Part model, mm, in its own coordinate system. A direction names the side the tool comes from. Coordinates: 2 decimals unless noted, no trailing zeros. Order: outer loops, then holes, each group sorted by start corner. A loop starts at its lowest first (then second) coordinate and runs counter-clockwise, first axis right, second up.
```python
from build123d import *

# Parameters (mm, degrees)
SKETCH1_W                 = 120
SKETCH1_H                 = 70
BOSS_EXTRUDE1_DEPTH       = 3
SKETCH6_W                 = 15
SKETCH6_H                 = 20
BOSS_EXTRUDE3_DEPTH       = 13
SKETCH7_W                 = 12.1
SKETCH7_H                 = 10.1
CUT_EXTRUDE3_DEPTH        = 71
SKETCH8_W                 = 15
SKETCH8_H                 = 4.3
BOSS_EXTRUDE4_DEPTH       = 2
SKETCH9_W                 = 1
SKETCH9_H                 = 6
CUT_EXTRUDE4_DEPTH        = 2
SKETCH10_W                = 3.5
SKETCH10_H                = 3
BOSS_EXTRUDE5_DEPTH       = 1.2
CHAMFER1_SIZE             = 1
CHAMFER1_OF_MIRROR3_SIZE  = 1
CUT_EXTRUDE5_REACH        = 18
SKETCH3_R                 = 1.625
SKETCH12_R                = 3
SKETCH12_R_2              = 1.625
BOSS_EXTRUDE7_DEPTH       = 4
CUT_EXTRUDE6_REACH        = 18
SKETCH11_R                = 1.625
SKETCH13_R                = 3
SKETCH13_R_2              = 1.625
BOSS_EXTRUDE8_DEPTH       = 4
SKETCH14_R                = 1.625
CUT_EXTRUDE7_DEPTH        = 4
SKETCH15_R                = 3.25
SKETCH15_R_2              = 1.625
SKETCH15_R_3              = 3
BOSS_EXTRUDE13_DEPTH      = 4
SKETCH17_W                = 5
SKETCH17_H                = 25
CUT_EXTRUDE8_DEPTH        = 4
SKETCH18_R                = 3
SKETCH18_R_2              = 1.625
BOSS_EXTRUDE14_DEPTH      = 4
FILLET2_R                 = 2
SKETCH19_R                = 1.625
CUT_EXTRUDE9_DEPTH        = 4
LPATTERN1_COUNT           = 2
LPATTERN1_PITCH           = 30
LPATTERN1_COL_COUNT       = 2
LPATTERN1_COL_PITCH       = 30
LPATTERN2_COUNT           = 4
LPATTERN2_PITCH           = 30
LPATTERN2_COPY_1_SKETCH_R = 1.625
LPATTERN2_COPY_1_DEPTH    = 4
LPATTERN2_COPY_2_SKETCH_R = 1.625
LPATTERN2_COPY_2_DEPTH    = 4
LPATTERN2_COPY_3_SKETCH_R = 1.625
LPATTERN2_COPY_3_DEPTH    = 4
LPATTERN2_COPY_4_SKETCH_R = 1.625
LPATTERN2_COPY_4_DEPTH    = 4
LPATTERN2_COPY_5_SKETCH_R = 1.625
LPATTERN2_COPY_5_DEPTH    = 4
LPATTERN2_COPY_6_SKETCH_R = 1.625
LPATTERN2_COPY_6_DEPTH    = 4


with BuildPart() as part:
    # Sketch1 → Boss-Extrude1 (new body)
    with BuildSketch(Plane(origin=(0, 0, 0), x_dir=(1, 0, 0), z_dir=(0, 1, 0))):
        Rectangle(SKETCH1_W, SKETCH1_H)
    extrude(amount=BOSS_EXTRUDE1_DEPTH)

    # Sketch6 → Boss-Extrude3 (add)
    with BuildSketch(Plane(origin=(0, 3, 0), x_dir=(1, 0, 0), z_dir=(0, 1, 0))):
        with Locations((-52.5, 25)):
            Rectangle(SKETCH6_W, SKETCH6_H)
        with Locations((-52.5, -25)):
            Rectangle(SKETCH6_W, SKETCH6_H)
    extrude(amount=BOSS_EXTRUDE3_DEPTH)

    # Sketch7 → Cut-Extrude3 (cut, through all)
    with BuildSketch(Plane(origin=(0, 0, -35), x_dir=(-1, 0, 0), z_dir=(0, 0, -1))):
        with Locations((52.55, 8.95)):
            Rectangle(SKETCH7_W, SKETCH7_H)
    extrude(amount=-CUT_EXTRUDE3_DEPTH, mode=Mode.SUBTRACT)

    # Sketch8 → Boss-Extrude4 (add)
    with BuildSketch(Plane(origin=(0, 3.9, 0), x_dir=(1, 0, 0), z_dir=(0, 1, 0))):
        with Locations((-52.5, -17.15)):
            Rectangle(SKETCH8_W, SKETCH8_H)
    boss_extrude4 = extrude(amount=BOSS_EXTRUDE4_DEPTH)

    # Mirror1: Boss-Extrude4 across plane
    add(boss_extrude4.mirror(Plane.XY))

    # Sketch9 → Cut-Extrude4 (cut)
    with BuildSketch(Plane(origin=(0, 16, 0), x_dir=(1, 0, 0), z_dir=(0, 1, 0))):
        with Locations((-54.75, 32)):
            Rectangle(SKETCH9_W, SKETCH9_H)
        with Locations((-50.25, 32)):
            Rectangle(SKETCH9_W, SKETCH9_H)
    cut_extrude4 = extrude(amount=-CUT_EXTRUDE4_DEPTH, mode=Mode.SUBTRACT)

    # Mirror2: Cut-Extrude4 across plane
    add(cut_extrude4.mirror(Plane.XY), mode=Mode.SUBTRACT)

    # Sketch10 → Boss-Extrude5 (add)
    with BuildSketch(Plane(origin=(0, 0, -35), x_dir=(-1, 0, 0), z_dir=(0, 0, -1))):
        with Locations((52.5, 14.5)):
            Rectangle(SKETCH10_W, SKETCH10_H)
    boss_extrude5 = extrude(amount=BOSS_EXTRUDE5_DEPTH)

    # Chamfer1
    chamfer1_edges = [part.edges().sort_by_distance(p)[0] for p in [
        (-52.5, 13, -36.2),
    ]]
    chamfer(chamfer1_edges, length=CHAMFER1_SIZE)

    # Mirror3: Boss-Extrude5 across plane
    add(boss_extrude5.mirror(Plane.XY))

    # Chamfer1 of Mirror3
    chamfer1_of_mirror3_edges = [part.edges().sort_by_distance(p)[0] for p in [
        (-52.5, 13, 36.2),
    ]]
    chamfer(chamfer1_of_mirror3_edges, length=CHAMFER1_OF_MIRROR3_SIZE)

    # Sketch3 → Cut-Extrude5 (cut, up to next)
    with BuildSketch(Plane.XZ, mode=Mode.PRIVATE) as cut_extrude5_sk1:
        with Locations((45, 18.875)):
            Circle(SKETCH3_R)
    cut_extrude5_tool1 = extrude(cut_extrude5_sk1.sketch, amount=-CUT_EXTRUDE5_REACH, mode=Mode.PRIVATE) & part.part
    add(cut_extrude5_tool1.solids().sort_by_distance((45, 0, 18.875))[0], mode=Mode.SUBTRACT)
    # Sketch3 → Cut-Extrude5 (cut, up to next)
    with BuildSketch(Plane.XZ, mode=Mode.PRIVATE) as cut_extrude5_sk2:
        with Locations((45, -18.875)):
            Circle(SKETCH3_R)
    cut_extrude5_tool2 = extrude(cut_extrude5_sk2.sketch, amount=-CUT_EXTRUDE5_REACH, mode=Mode.PRIVATE) & part.part
    add(cut_extrude5_tool2.solids().sort_by_distance((45, 0, -18.875))[0], mode=Mode.SUBTRACT)

    # Sketch12 → Boss-Extrude7 (add)
    with BuildSketch(Plane(origin=(0, 3, 0), x_dir=(1, 0, 0), z_dir=(0, 1, 0))):
        with Locations((45, 18.875)):
            Circle(SKETCH12_R)
        with Locations((45, 18.875)):
            Circle(SKETCH12_R_2, mode=Mode.SUBTRACT)
    boss_extrude7 = extrude(amount=BOSS_EXTRUDE7_DEPTH)

    # Mirror4: Boss-Extrude7 across plane
    add(boss_extrude7.mirror(Plane.XY))

    # Sketch11 → Cut-Extrude6 (cut, up to next)
    with BuildSketch(Plane.XZ, mode=Mode.PRIVATE) as cut_extrude6_sk1:
        with Locations((20, 0)):
            Circle(SKETCH11_R)
    cut_extrude6_tool1 = extrude(cut_extrude6_sk1.sketch, amount=-CUT_EXTRUDE6_REACH, mode=Mode.PRIVATE) & part.part
    add(cut_extrude6_tool1.solids().sort_by_distance((20, 0, 0))[0], mode=Mode.SUBTRACT)

    # Sketch13 → Boss-Extrude8 (add)
    with BuildSketch(Plane(origin=(0, 3, 0), x_dir=(1, 0, 0), z_dir=(0, 1, 0))):
        with Locations((20, 0)):
            Circle(SKETCH13_R)
        with Locations((20, 0)):
            Circle(SKETCH13_R_2, mode=Mode.SUBTRACT)
    extrude(amount=BOSS_EXTRUDE8_DEPTH)

    # Sketch14 → Cut-Extrude7 (cut, through all)
    with BuildSketch(Plane(origin=(0, 3, 0), x_dir=(1, 0, 0), z_dir=(0, 1, 0))):
        with Locations((-42, 18.5)):
            Circle(SKETCH14_R)
        with Locations((-42, -18.5)):
            Circle(SKETCH14_R)
        with Locations((-5, 18.5)):
            Circle(SKETCH14_R)
        with Locations((-5, -18.5)):
            Circle(SKETCH14_R)
    extrude(amount=-CUT_EXTRUDE7_DEPTH, mode=Mode.SUBTRACT)

    # Sketch15 → Boss-Extrude13 (add)
    with BuildSketch(Plane(origin=(0, 3, 0), x_dir=(1, 0, 0), z_dir=(0, 1, 0))):
        with Locations((-42, 18.5)):
            Circle(SKETCH15_R)
        with Locations((-42, 18.5)):
            Circle(SKETCH15_R_2, mode=Mode.SUBTRACT)
        with Locations((-5, 18.5)):
            Circle(SKETCH15_R_3)
        with Locations((-5, 18.5)):
            Circle(SKETCH15_R_2, mode=Mode.SUBTRACT)
        with Locations((-5, -18.5)):
            Circle(SKETCH15_R_3)
        with Locations((-5, -18.5)):
            Circle(SKETCH15_R_2, mode=Mode.SUBTRACT)
        with Locations((-42, -18.5)):
            Circle(SKETCH15_R)
        with Locations((-42, -18.5)):
            Circle(SKETCH15_R_2, mode=Mode.SUBTRACT)
    extrude(amount=BOSS_EXTRUDE13_DEPTH)

    # Sketch17 → Cut-Extrude8 (cut, through all)
    with BuildSketch(Plane(origin=(0, 3, 0), x_dir=(1, 0, 0), z_dir=(0, 1, 0))):
        with Locations((32.5, 0)):
            Rectangle(SKETCH17_W, SKETCH17_H)
    extrude(amount=-CUT_EXTRUDE8_DEPTH, mode=Mode.SUBTRACT)

    # Sketch18 → Boss-Extrude14 (add)
    with BuildSketch(Plane(origin=(0, 16, 0), x_dir=(1, 0, 0), z_dir=(0, 1, 0))):
        with Locations((-52.5, 22.5)):
            Circle(SKETCH18_R)
        with Locations((-52.5, 22.5)):
            Circle(SKETCH18_R_2, mode=Mode.SUBTRACT)
    boss_extrude14 = extrude(amount=BOSS_EXTRUDE14_DEPTH)

    # Mirror5: Boss-Extrude14 across plane
    add(boss_extrude14.mirror(Plane.XY))

    # Fillet2
    fillet2_edges = [part.edges().sort_by_distance(p)[0] for p in [
        (30, 1.5, 12.5),
        (30, 1.5, -12.5),
        (35, 1.5, -12.5),
        (35, 1.5, 12.5),
        (60, 1.5, -35),
        (60, 1.5, 35),
    ]]
    fillet(fillet2_edges, radius=FILLET2_R)

    # Sketch19 → Cut-Extrude9 (cut, through all)
    with BuildSketch(Plane(origin=(0, 3, 0), x_dir=(1, 0, 0), z_dir=(0, 1, 0))):
        with Locations((55, 0)):
            Circle(SKETCH19_R)
    cut_extrude9 = extrude(amount=-CUT_EXTRUDE9_DEPTH, mode=Mode.SUBTRACT)

    # LPattern1: Cut-Extrude9 ×2
    with Locations(*[(0, 0, i * LPATTERN1_PITCH) for i in range(1, LPATTERN1_COUNT)]):
        add(cut_extrude9, mode=Mode.SUBTRACT)

    # LPattern1 col: Cut-Extrude9 ×2
    with Locations(*[(0, 0, -i * LPATTERN1_COL_PITCH) for i in range(1, LPATTERN1_COL_COUNT)]):
        add(cut_extrude9, mode=Mode.SUBTRACT)

    # LPattern2: Cut-Extrude9 ×4
    with Locations(*[(-i * LPATTERN2_PITCH, 0, 0) for i in range(1, LPATTERN2_COUNT)]):
        add(cut_extrude9, mode=Mode.SUBTRACT)

    # LPattern2 copy 1 sketch → LPattern2 copy 1 (cut, through all)
    with BuildSketch(Plane(origin=(-30, 3, 30), x_dir=(1, 0, 0), z_dir=(0, 1, 0))):
        with Locations((55, 0)):
            Circle(LPATTERN2_COPY_1_SKETCH_R)
    extrude(amount=-LPATTERN2_COPY_1_DEPTH, mode=Mode.SUBTRACT)

    # LPattern2 copy 2 sketch → LPattern2 copy 2 (cut, through all)
    with BuildSketch(Plane(origin=(-60, 3, 30), x_dir=(1, 0, 0), z_dir=(0, 1, 0))):
        with Locations((55, 0)):
            Circle(LPATTERN2_COPY_2_SKETCH_R)
    extrude(amount=-LPATTERN2_COPY_2_DEPTH, mode=Mode.SUBTRACT)

    # LPattern2 copy 3 sketch → LPattern2 copy 3 (cut, through all)
    with BuildSketch(Plane(origin=(-90, 3, 30), x_dir=(1, 0, 0), z_dir=(0, 1, 0))):
        with Locations((55, 0)):
            Circle(LPATTERN2_COPY_3_SKETCH_R)
    extrude(amount=-LPATTERN2_COPY_3_DEPTH, mode=Mode.SUBTRACT)

    # LPattern2 copy 4 sketch → LPattern2 copy 4 (cut, through all)
    with BuildSketch(Plane(origin=(-30, 3, -30), x_dir=(1, 0, 0), z_dir=(0, 1, 0))):
        with Locations((55, 0)):
            Circle(LPATTERN2_COPY_4_SKETCH_R)
    extrude(amount=-LPATTERN2_COPY_4_DEPTH, mode=Mode.SUBTRACT)

    # LPattern2 copy 5 sketch → LPattern2 copy 5 (cut, through all)
    with BuildSketch(Plane(origin=(-60, 3, -30), x_dir=(1, 0, 0), z_dir=(0, 1, 0))):
        with Locations((55, 0)):
            Circle(LPATTERN2_COPY_5_SKETCH_R)
    extrude(amount=-LPATTERN2_COPY_5_DEPTH, mode=Mode.SUBTRACT)

    # LPattern2 copy 6 sketch → LPattern2 copy 6 (cut, through all)
    with BuildSketch(Plane(origin=(-90, 3, -30), x_dir=(1, 0, 0), z_dir=(0, 1, 0))):
        with Locations((55, 0)):
            Circle(LPATTERN2_COPY_6_SKETCH_R)
    extrude(amount=-LPATTERN2_COPY_6_DEPTH, mode=Mode.SUBTRACT)


solid = part.part
```
(1) Drop flat-ended pins along their axis: pin 1 (7.5 mm diameter, centred on x = -49, z = -25, fed in from +Y); pin 2 (2 mm diameter, centred on x = -2, y = 3, fed in from +Z); pin 3 (3 mm diameter, centred on y = 6.5, z = 23, fed in from +X); pin 4 (3 mm diameter, centred on x = 44.5, z = -20, fed in from +Y). Give the stop position or say it passes through.
(2) Tool access for faces 4 (the face through (53.377, 1.521, -0.071)), 5 (the face through (-58.6, 9, 25)), 6 (the face through (-1, 3, 0)): list every direction of +Z, -Z, +X, -X, +Y, -Y with a clear straight run to the whole face (end or side of a thin tool).
(3) Slice it at B-B, the plane x = -35. Give the cut face in (y, z) (3 decimals).
(4) Probe line 1 (Z direction, x = -42, y = 6.1) (3 decimals); line 2 (Z direction, x = 55, y = 1.6) (3 decimals); line 3 (X direction, y = 15.25, z = -31). List the from-to ranges inside material, lowest first.
(5) Slice it at A-A, the plane z = 0. State how many separate pieces and enclosed holes the cut face has, then the cut area to 3 significant figures.
(6) Slice it at D-D, the plane z = 9. Give the cut face in (x, y).
(7) Slice it at C-C, the plane y = 18.75. Give the cut face in (x, z) (3 decimals), then the cut area to 3 significant figures.
(8) Pull direction Z, two halves, no side cores. Call faces 1 (the face through (-46.5, 9, -25)), 2 (the face through (-5.65, 4.97, 21.43)), 3 (the face through (-36.623, 1.521, -0.071)): +Z half, -Z half, draft (parallel to the pull), parting line (faces both ways), or undercut.
Here are the results:
1. pin 1: stops at y = 20
1. pin 2: stops at z = 35
1. pin 3: stops at x = 46.45
1. pin 4: stops at y = 7
2. face 4: +Y, -Y
2. face 5: +Z
2. face 6: +Y
3. outline: (0, -35) - (3, -35) - (3, -31.625) - (0, -31.625) - close; (0, -28.375) - (3, -28.375) - (3, -1.625) - (0, -1.625) - close; (0, 1.625) - (3, 1.625) - (3, 28.375) - (0, 28.375) - close; (0, 31.625) - (3, 31.625) - (3, 35) - (0, 35) - close
4. line 1: z = -21.75 to -20.125, -16.875 to -15.25, 15.25 to 16.875, 20.125 to 21.75
4. line 2: z = -35 to -31.625, -28.375 to -1.625, 1.625 to 28.375, 31.625 to 35
4. line 3: x = -60 to -55.25, -54.25 to -50.75, -49.75 to -45
5. separate pieces: 7
5. enclosed holes: 0
5. area: 307 mm2
6. outline: (-60, 0) - (30, 0) - (30, 3) - (-60, 3) - close; (35, 0) - (60, 0) - (60, 3) - (35, 3) - close
7. outline: circle Ø6 at (-52.5, -22.5); circle Ø6 at (-52.5, 22.5); hole circle Ø3.25 at (-52.5, -22.5); hole circle Ø3.25 at (-52.5, 22.5)
7. area: 40.0 mm2
8. face 1: draft
8. face 2: undercut
8. face 3: undercut
